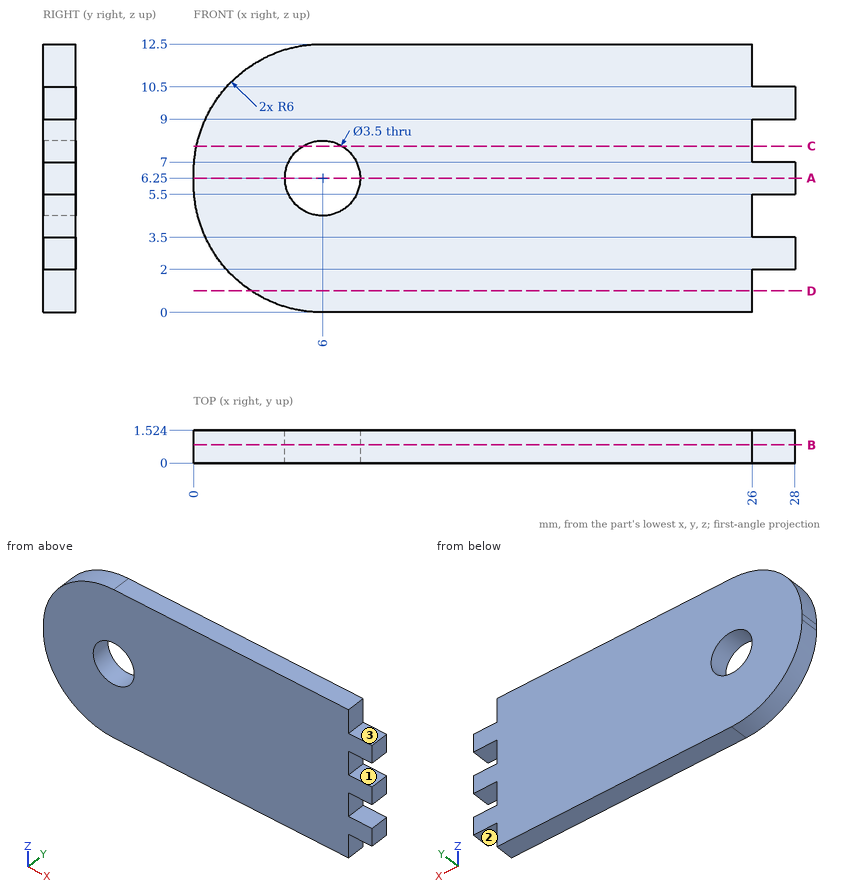
Geometry: see drawing. Coordinates: mm, zero at the bounding-box minimum. A direction names the side the tool comes from. Round coordinates to 2 decimals unless told otherwise and drop trailing zeros. Loops run counter-clockwise (first coordinate to the right, second up) from the corner with the lowest first, then second, coordinate; pieces in that order, holes last.
(1) Section query D-D (z = 1). Output: boundary loops of the cut face in (x, y), and give its area (3 significant figures).
From the geometry:
outline: (2.68, 0) - (26, 0) - (26, 1.52) - (2.68, 1.52) - close
area: 35.5 mm2
(2) Section query A-A (z = 6.25). Output: boundary loops of the cut face in (x, y), and give its area (3 significant figures).
From the geometry:
outline: (0, 0) - (4.25, 0) - (4.25, 1.52) - (0, 1.52) - close; (7.75, 0) - (28, 0) - (28, 1.52) - (7.75, 1.52) - close
area: 37.3 mm2
(3) Section query C-C (z = 7.75). Output: boundary loops of the cut face in (x, y), and give its area (3 significant figures).
From the geometry:
outline: (0.13, 0) - (5.1, 0) - (5.1, 1.52) - (0.13, 1.52) - close; (6.9, 0) - (26, 0) - (26, 1.52) - (6.9, 1.52) - close
area: 36.7 mm2
(4) Contact query for flat-ended pins moving along their axis: pin 1 Ø0.8 at (x, y) = (27, 0.5) entering from -Z; pin 2 Ø0.5 at (x, y) = (26.5, 0.5) entering from +Z; pin 3 Ø0.8 at (y, z) = (0.5, 4) entering from +X. Output: stop coordinate, or through.
From the geometry:
pin 1: stops at z = 2
pin 2: stops at z = 10.5
pin 3: stops at x = 26
(5) Material intervals for probe 1 along Z at (x, y) = (6.5, 0.15); probe 2 along X at (y, z) = (0.5, 9.5); probe 3 along X at (y, z) = (1.3, 1), sorted ascending.
From the geometry:
probe 1: z = 0 to 4.57, 7.93 to 12.5
probe 2: x = 0.8 to 28
probe 3: x = 2.68 to 26
(6) Section query B-B (y = 0.85). Output: boundary loops of the cut face in (x, z).
From the geometry:
outline: (0, 6) arc R6 ccw to (6, 0) - (26, 0) - (26, 2) - (28, 2) - (28, 3.5) - (26, 3.5) - (26, 5.5) - (28, 5.5) - (28, 7) - (26, 7) - (26, 9) - (28, 9) - (28, 10.5) - (26, 10.5) - (26, 12.5) - (6, 12.5) arc R6 ccw to (0, 6.5) - close; hole circle Ø3.5 at (6, 6.25)
(7) Access query for the marked faces 1, 2 and 3. Directions: +Z, -Z, +X, -X, +Y, -Y. A direction counts if a zero-diameter tool reaches every point of the face in a straight line with its end or side. Return the directions, or none.
From the geometry:
face 1: +X, +Y, -Y
face 2: -Z, +X, +Y, -Y
face 3: +Z, +X, +Y, -Y
